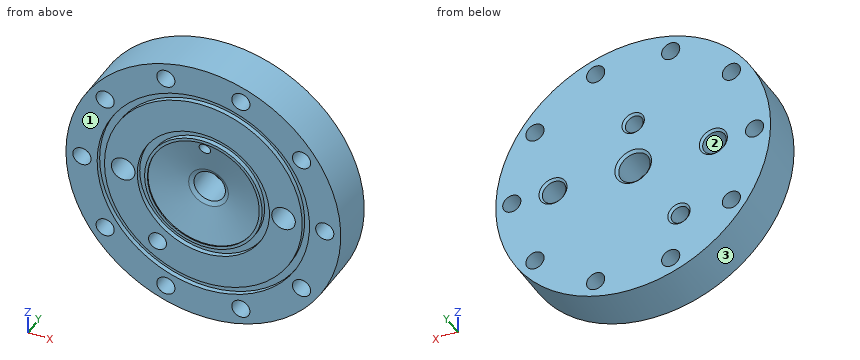
```python
from build123d import *

# Parameters (mm, degrees)
F_3_4_16_TAPPED_HOLE1_D            = 17.4625
F_3_4_16_TAPPED_HOLE1_CSINK_D      = 20.32
F_3_4_16_TAPPED_HOLE1_CSINK_ANGLE  = 90
F_9_16_18_TAPPED_HOLE1_D           = 13.09624
F_9_16_18_TAPPED_HOLE1_CSINK_D     = 15.5575
F_9_16_18_TAPPED_HOLE1_CSINK_ANGLE = 90
F_3_8_CLEARANCE_HOLE2_D            = 10.0838
CIRPATTERN1_COUNT                  = 10
F_7_16_20_TAPPED_HOLE1_D           = 9.92124
F_7_16_20_TAPPED_HOLE1_DEPTH       = 14.799358796
F_7_16_20_TAPPED_HOLE1_CSINK_D     = 12.3825
F_7_16_20_TAPPED_HOLE1_CSINK_ANGLE = 90
F_7_16_20_TAPPED_HOLE1_TIP         = 2.980641204
F_7_16_20_TAPPED_HOLE2_D           = 9.92124
F_7_16_20_TAPPED_HOLE2_CSINK_D     = 12.3825
F_7_16_20_TAPPED_HOLE2_CSINK_ANGLE = 90
F_1_4_0_25_DIAMETER_HOLE2_D        = 6.35
F_1_4_0_25_DIAMETER_HOLE2_DEPTH    = 72.260267535
F_1_4_0_25_DIAMETER_HOLE2_TIP      = 1.907732465


with BuildPart() as part:
    # Sketch1 → Revolve1 (revolve)
    with BuildSketch(Plane.XY):
        Polygon((0, 0), (-76.2, 0), (-76.2, -25.4), (-58.8899, -25.4), (-58.8899, -22.7076), (-54.8259, -22.7076), (-54.8259, -25.4), (-36.6649, -25.4), (-36.6649, -22.7076), (-32.6009, -22.7076), (-32.6009, -25.4), (-31.0134, -25.4), (-31.0134, -24.765), (-10.9982, -19.812), (0, -13.462186269), align=None)
    revolve(axis=Axis((0, 0, 0), (0, -1, 0)))

    # 3/4-16 Tapped Hole1 (through all)
    with Locations(Plane(origin=(0, 0, 0), x_dir=(1, 0, 0), z_dir=(0, 1, 0))):
        with Locations((0, 0)):
            CounterSinkHole(F_3_4_16_TAPPED_HOLE1_D / 2, F_3_4_16_TAPPED_HOLE1_CSINK_D / 2, counter_sink_angle=F_3_4_16_TAPPED_HOLE1_CSINK_ANGLE)

    # 9/16-18 Tapped Hole1 (through all)
    with Locations(Plane(origin=(0, 0, 0), x_dir=(1, 0, 0), z_dir=(0, 1, 0))):
        with Locations((-44.45, 0), (44.45, 0)):
            CounterSinkHole(F_9_16_18_TAPPED_HOLE1_D / 2, F_9_16_18_TAPPED_HOLE1_CSINK_D / 2, counter_sink_angle=F_9_16_18_TAPPED_HOLE1_CSINK_ANGLE)

    # 3/8 Clearance Hole2 (through all)
    with Locations(Plane(origin=(67.31, 0, 0), x_dir=(0, 0, 1), z_dir=(0, 1, 0))):
        with Locations((0, 0)):
            f_3_8_clearance_hole2 = Hole(F_3_8_CLEARANCE_HOLE2_D / 2)

    # CirPattern1: 3/8 Clearance Hole2 ×10 about axis
    cirpattern1_axis = Axis((0, 0, 0), (0, 1, 0))
    for i in range(1, CIRPATTERN1_COUNT):
        add(f_3_8_clearance_hole2.rotate(cirpattern1_axis, i * 360 / CIRPATTERN1_COUNT), mode=Mode.SUBTRACT)

    # 7/16-20 Tapped Hole1
    with Locations(Plane(origin=(0, 0, 26.67), x_dir=(1, 0, 0), z_dir=(0, 1, 0))):
        with Locations((0, 0)):
            CounterSinkHole(F_7_16_20_TAPPED_HOLE1_D / 2, F_7_16_20_TAPPED_HOLE1_CSINK_D / 2, depth=F_7_16_20_TAPPED_HOLE1_DEPTH, counter_sink_angle=F_7_16_20_TAPPED_HOLE1_CSINK_ANGLE)
            with Locations((0, 0, -(F_7_16_20_TAPPED_HOLE1_DEPTH + F_7_16_20_TAPPED_HOLE1_TIP / 2))):  # 118° drill point
                Cone(0, F_7_16_20_TAPPED_HOLE1_D / 2, F_7_16_20_TAPPED_HOLE1_TIP, mode=Mode.SUBTRACT)

    # 7/16-20 Tapped Hole2 (through all)
    with Locations(Plane(origin=(-25.4, 0, -38.1), x_dir=(0, 0, 1), z_dir=(0, 1, 0))):
        with Locations((0, 0)):
            CounterSinkHole(F_7_16_20_TAPPED_HOLE2_D / 2, F_7_16_20_TAPPED_HOLE2_CSINK_D / 2, counter_sink_angle=F_7_16_20_TAPPED_HOLE2_CSINK_ANGLE)

    # 1/4 (0.25) Diameter Hole2
    with Locations(Plane(origin=(0, 0, 0), x_dir=(1, 0, 0), z_dir=(0, 1, 0))):
        with Locations((0, -26.67)):
            Hole(F_1_4_0_25_DIAMETER_HOLE2_D / 2, depth=F_1_4_0_25_DIAMETER_HOLE2_DEPTH)
            with Locations((0, 0, -(F_1_4_0_25_DIAMETER_HOLE2_DEPTH + F_1_4_0_25_DIAMETER_HOLE2_TIP / 2))):  # 118° drill point
                Cone(0, F_1_4_0_25_DIAMETER_HOLE2_D / 2, F_1_4_0_25_DIAMETER_HOLE2_TIP, mode=Mode.SUBTRACT)


solid = part.part
```
Check sheet for the modelled part. Datum: model origin and axes. Units: mm. Face numbers are marked on the shaded views. Coordinates: 2 decimals unless noted, no trailing zeros. Order: outer loops, then holes, each group sorted by start corner. A loop starts at its lowest first (then second) coordinate and runs counter-clockwise, first axis right, second up. Notation, with made-up numbers: (12, 37) -> (54, 37) arc R7 cw to (54, 46) -> close; hole circle Ø8 at (-12, 34). An arc over 180 degrees is marked (long way). Write item = value, one per line. Start each with the question number.
1) Cross-section at D-D (x = 67.31). Enter the section's corners in (y, z), then the cut area to 3 significant figures.
2) Cross-section at A-A (x = 44.45). Enter the section's corners in (y, z).
3) Go/stop test with flat-tipped pins: P1, Ø1, axis at y = -21, z = 16, coming from the +X side; P2, Ø10, axis at x = 14, y = -22, coming from the +Z side; P3, Ø4, axis at x = 43, y = -4, coming from the +Z side. Record where each tip stops, or that it passes through.
4) Material ranges on L1, parallel to Z at x = -53, y = -22.5; L2, parallel to X at y = -21.75, z = 44; L3, parallel to X at y = -11.5, z = 68, recorded low to high.
5) Mould release check, pull along X, two halves, no side actions. Record for the marked faces 1, 2 and 3: +X half, -X half, draft (parallel to the pull), parting line (faces both ways), or undercut.
6) Cross-section at B-B (y = -4). State how many separate pieces and enclosed holes the cut face has, then the cut area to 3 significant figures.
Ans:
q1.outline = (-25.4, -35.72) -> (0, -35.72) -> (0, -5.04) -> (-25.4, -5.04) -> close; (-25.4, 5.04) -> (0, 5.04) -> (0, 35.72) -> (-25.4, 35.72) -> close
q1.area = 1,560 mm²
q2.outline = (-25.4, -61.89) -> (0, -61.89) -> (0, -7.78) -> (-1.23, -6.55) -> (-25.4, -6.55) -> (-25.4, -32.09) -> (-22.71, -32.09) -> (-22.71, -38.63) -> (-25.4, -38.63) -> close; (-25.4, 6.55) -> (-1.23, 6.55) -> (0, 7.78) -> (0, 61.89) -> (-25.4, 61.89) -> (-25.4, 38.63) -> (-22.71, 38.63) -> (-22.71, 32.09) -> (-25.4, 32.09) -> close
q3.P1 = 74.61
q3.P2 = 75.67
q3.P3 = 64.23
q4.L1 = -54.75 to -44.39, -34.74 to 34.74, 44.39 to 54.75
q4.L2 = -62.21 to -56.85, -52.06 to 52.06, 56.85 to 62.21
q4.L3 = -34.39 to -23.89, -17.71 to 17.71, 23.89 to 34.39
q5.face_1 = draft
q5.face_2 = undercut
q5.face_3 = parting line
q6.separate_pieces = 1
q6.enclosed_holes = 15
q6.area = 16,800 mm²
